Model file for the job. Use its own axes, mm. A direction names the side the tool comes from. Round coordinates to 2 decimals unless told otherwise and drop trailing zeros. Write each loop counter-clockwise with the first axis right and the second up, starting at its lowest first coordinate (ties: lowest second). Pieces come first, ordered by that corner, then holes. Notation, with made-up numbers: (45, -5) - (80, -5) arc R22 cw to (80, 19) - close; hole circle Ø5 at (37.5, 44.5). An arc over 180 degrees is marked (long way). Answer as a JSON object with one key per item and string values. Group by question number.
from build123d import *

# Parameters (mm, degrees)
F0_W     = 15
F0_H     = 60
F1_DEPTH = 50
F2_DEPTH = 30
F3_SIZE2 = 10
F3_SIZE  = 20


with BuildPart() as f1:
    # F0 (on Front) → F1 (new body)
    with BuildSketch(Plane.XZ):
        with Locations((7.5, 30)):
            Rectangle(F0_W, F0_H)
        Polygon((15, 60), (15, 0), (90, 0), (90, 30), (30, 60), align=None)
        Polygon((90, 30), (90, 0), (110, 0), (110, 20), align=None)
    extrude(amount=-F1_DEPTH)

    # F0 (on Front) → F2 (cut)
    with BuildSketch(Plane.XZ):
        Polygon((15, 60), (15, 0), (90, 0), (90, 30), (30, 60), align=None)
    extrude(amount=-F2_DEPTH, mode=Mode.SUBTRACT)

    # F3
    f3_edges = [f1.edges().sort_by_distance(p)[0] for p in [
        (7.5, 0, 60),
    ]]
    f3_side = f1.faces().sort_by_distance((11.785714, 29.285714, 60))[0]
    chamfer(f3_edges, length=F3_SIZE, length2=F3_SIZE2, reference=f3_side)


solid = f1.part
(1) Pull direction X, two halves, no side cores. Call faces 1 (the flat face through (44, 30, 24)), 2 (the flat face through (79.4, 35.8, 35.3)), 3 (the flat face through (15, 15, 30)), 4 (the flat face through (42, 50, 24)): pulls with the +X half, pulls with the -X half, needs draft (parallel to the pull), parting line crosses it, or undercut.
(2) Flat gauge pins, fed straight in: pin 1 (3 mm diameter, centred on y = 41.5, z = 34.5, fed in from +X); pin 2 (8 mm diameter, centred on y = 44, z = 47, fed in from +X). Where does each tip first touch, or does it go through?
(3) Slice it at C-C (y = 4). Write the cut outline in (x, z), then the cut area to 3 significant figures.
(4) Slice it at B-B (z = 12.5). Write the cut outline in (x, y).
(5) Slice it at D-D (x = 84.5). Write the cut outline in (y, z), then the cut area to 3 significant figures.
(6) 3-axis set-ups, long thin cutter, end or side, ignore diameter. For faces 5 (the flat face through (90, 15, 15)), 6 (the flat face through (7, 0, 25)): which of +Z, -Z, +X, -X, +Y, -Y reach the whole face in a straight line?
(7) Drill centre lines: line 1 (X direction, y = 15.5, z = 8); line 2 (X direction, y = 27, z = 33); line 3 (Y direction, x = 60, z = 5.5). Where is each one in solid material? Low to high. Write a range as from..to.
(8) Slice it at A-A (y = 11.5). Write the cut outline in (x, z), then the cut area to 3 significant figures.
Answer:
{
 "1": {"face 1": "undercut", "face 2": "pulls with the +X half", "face 3": "undercut", "face 4": "needs draft"},
 "2": {"pin 1": "x = 84", "pin 2": "x = 64"},
 "3": {"outline": "(0, 0) - (15, 0) - (15, 52) - (0, 52) - close; (90, 0) - (110, 0) - (110, 20) - (90, 30) - close", "area": "1,280 mm²"},
 "4": {"outline": "(0, 0) - (15, 0) - (15, 30) - (90, 30) - (90, 0) - (110, 0) - (110, 50) - (0, 50) - close"},
 "5": {"outline": "(30, 0) - (50, 0) - (50, 32.75) - (30, 32.75) - close", "area": "655 mm²"},
 "6": {"face 5": "+Z, -Z, -Y", "face 6": "+Z, -Z, +X, -X, -Y"},
 "7": {"line 1": "0..15, 90..110", "line 2": "0..15", "line 3": "30..50"},
 "8": {"outline": "(0, 0) - (15, 0) - (15, 55.75) - (0, 55.75) - close; (90, 0) - (110, 0) - (110, 20) - (90, 30) - close", "area": "1,340 mm²"}
}
